Could you check a few things on this model? Use its own coordinates, in mm. Round coordinates to 2 decimals unless told otherwise and drop trailing zeros. Loops run counter-clockwise (first coordinate to the right, second up) from the corner with the lowest first, then second, coordinate; pieces in that order, holes last. Notation, with made-up numbers: (40.5, -29.75) -> (67.5, -29.75) arc R14 cw to (67.5, -4.75) -> close; hole circle Ø3 at (12, 40.5). An arc over 180 degrees is marked (long way). One line per item, written item: value.
Autodesk Inventor part; units mm, degrees
ref_plane "Startebene" through (0, 0, 0) normal (0, 0, 1) x (1, 0, 0)
ref_plane "Endebene" through (0, 0, 320) normal (0, 0, 1) x (1, 0, 0)
ref_plane "Startebene1" through (0, 0, 0) normal (0, 0, 1) x (1, 0, 0)
ref_plane "Startebene" through (0, 0, 0) normal (0, 0, 1) x (1, 0, 0)
ref_plane "Endebene" through (0, 0, 320) normal (0, 0, 1) x (1, 0, 0)
ref_plane "Startebene1" through (0, 0, 0) normal (0, 0, 1) x (1, 0, 0)
ref_plane "Endebene1" through (0, 0, 80) normal (0, 0, 1) x (1, 0, 0)
ref_plane "Startebene2" through (0, 0, 10) normal (0, 0, 1) x (1, 0, 0)
ref_plane "Endebene2" through (0, 0, 70) normal (0, 0, 1) x (1, 0, 0)
sketch "Skizze" plane through (0, 0, 0) normal (0, 0, 1) x (1, 0, 0)
  line L0 (-10, 9) -> (-10, 3.3)
  arc A0 (-10, 3.3) -> (-9.7, 3) centre (-9.7, 3.3) ccw
  line L1 (-9.7, 3) -> (-8, 3)
  line L2 (-8, 3) -> (-8, 6)
  line L3 (-8, 6) -> (-7.0607, 6)
  line L4 (-7.0607, 6) -> (-4, 2.9393)
  line L5 (-4, 2.9393) -> (-4, 0.3)
  line L6 (-4, 0.3) -> (-3.7, 0)
  line L7 (-3.7, 0) -> (-4, -0.3)
  line L8 (-4, -0.3) -> (-4, -2.9393)
  line L9 (-4, -2.9393) -> (-7.0607, -6)
  line L10 (-7.0607, -6) -> (-8, -6)
  line L11 (-8, -6) -> (-8, -3)
  line L12 (-8, -3) -> (-9.7, -3)
  arc A1 (-9.7, -3) -> (-10, -3.3) centre (-9.7, -3.3) ccw
  line L13 (-10, -3.3) -> (-10, -9)
  arc A2 (-10, -9) -> (-9, -10) centre (-9, -9) ccw
  line L14 (-9, -10) -> (-3.3, -10)
  arc A3 (-3.3, -10) -> (-3, -9.7) centre (-3.3, -9.7) ccw
  line L15 (-3, -9.7) -> (-3, -8)
  line L16 (-3, -8) -> (-6, -8)
  line L17 (-6, -8) -> (-6, -7.0607)
  line L18 (-6, -7.0607) -> (-2.9393, -4)
  line L19 (-2.9393, -4) -> (-0.3, -4)
  line L20 (-0.3, -4) -> (0, -3.7)
  line L21 (0, -3.7) -> (0.3, -4)
  line L22 (0.3, -4) -> (2.9393, -4)
  line L23 (2.9393, -4) -> (6, -7.0607)
  line L24 (6, -7.0607) -> (6, -8)
  line L25 (6, -8) -> (3, -8)
  line L26 (3, -8) -> (3, -9.7)
  arc A4 (3, -9.7) -> (3.3, -10) centre (3.3, -9.7) ccw
  line L27 (3.3, -10) -> (9, -10)
  arc A5 (9, -10) -> (10, -9) centre (9, -9) ccw
  line L28 (10, -9) -> (10, -3.3)
  arc A6 (10, -3.3) -> (9.7, -3) centre (9.7, -3.3) ccw
  line L29 (9.7, -3) -> (8, -3)
  line L30 (8, -3) -> (8, -6)
  line L31 (8, -6) -> (7.0607, -6)
  line L32 (7.0607, -6) -> (4, -2.9393)
  line L33 (4, -2.9393) -> (4, -0.3)
  line L34 (4, -0.3) -> (3.7, 0)
  line L35 (3.7, 0) -> (4, 0.3)
  line L36 (4, 0.3) -> (4, 2.9393)
  line L37 (4, 2.9393) -> (7.0607, 6)
  line L38 (7.0607, 6) -> (8, 6)
  line L39 (8, 6) -> (8, 3)
  line L40 (8, 3) -> (9.7, 3)
  arc A7 (9.7, 3) -> (10, 3.3) centre (9.7, 3.3) ccw
  line L41 (10, 3.3) -> (10, 9)
  arc A8 (10, 9) -> (9, 10) centre (9, 9) ccw
  line L42 (9, 10) -> (3.3, 10)
  arc A9 (3.3, 10) -> (3, 9.7) centre (3.3, 9.7) ccw
  line L43 (3, 9.7) -> (3, 8)
  line L44 (3, 8) -> (6, 8)
  line L45 (6, 8) -> (6, 7.0607)
  line L46 (6, 7.0607) -> (2.9393, 4)
  line L47 (2.9393, 4) -> (0.3, 4)
  line L48 (0.3, 4) -> (0, 3.7)
  line L49 (0, 3.7) -> (-0.3, 4)
  line L50 (-0.3, 4) -> (-2.9393, 4)
  line L51 (-2.9393, 4) -> (-6, 7.0607)
  line L52 (-6, 7.0607) -> (-6, 8)
  line L53 (-6, 8) -> (-3, 8)
  line L54 (-3, 8) -> (-3, 9.7)
  arc A10 (-3, 9.7) -> (-3.3, 10) centre (-3.3, 9.7) ccw
  line L55 (-3.3, 10) -> (-9, 10)
  arc A11 (-9, 10) -> (-10, 9) centre (-9, 9) ccw
  circle A12 centre (0, 0) radius 2.75
  dimension "d2" = 5.5
  dimension "d3" = 10
  dimension "d4" = 10
  dimension "d5" = 5.7
  dimension "d6" = 5.7
  dimension "d7" = 1.7
  dimension "d8" = 3
  dimension "d9" = 0.3
  dimension "d10" = 90
  dimension "d11" = 45
  dimension "d12" = 45
  dimension "d13" = 45
  dimension "d14" = 90
  dimension "d15" = 90
  dimension "d16" = 45
  dimension "d17" = 45
  dimension "d18" = 45
  dimension "d19" = 45
  dimension "d20" = 90
  dimension "d21" = 90
  dimension "d22" = 45
  dimension "d23" = 45
  dimension "d24" = 90
  dimension "d25" = 90
  dimension "d26" = 90
  dimension "d27" = 90
  dimension "d28" = 90
  dimension "d29" = 90
  dimension "d30" = 90
  dimension "d31" = 90
  dimension "d32" = 90
  dimension "d33" = 90
  dimension "d34" = 90
  dimension "d35" = 90
  dimension "d36" = 90
  dimension "d37" = 90
  dimension "d38" = 90
  dimension "d39" = 4
  dimension "d40" = 6
  dimension "d41" = 13
  dimension "d42" = 14
  dimension "d43" = 16
  dimension "d44" = 18
  dimension "d45" = 3
  dimension "d46" = 9
  dimension "d47" = 7
  dimension "d48" = 1
  dimension "d49" = 7
  dimension "d50" = 1.5
  dimension "d51" = 1.8663
  dimension "d52" = 3.3663
  dimension "d53" = 1.5
  dimension "d54" = 1.8663
  dimension "d55" = 3.3663
  dimension "d56" = 4
  dimension "d57" = 10.8187
  dimension "d58" = 1.9092
  dimension "d59" = 5
  dimension "d60" = 13
  dimension "d61" = 13
  dimension "d62" = 16.0513
  dimension "d63" = 3.3234
  dimension "d64" = 14
  dimension "d65" = 12.685
extrude "Körper" add sketch "Skizze" along normal up to surface (60 mm away) from surface at 10
sketch "Skizze13" plane through (0, 0, 0) normal (0, 0, 1) x (1, 0, 0)
  line L0 (0, 0) -> (10, 0)
ref_plane "Arbeitsebene12" through (0, 0, 0) normal (0, -1, 0) x (1, 0, 0)
sketch "Skizze14" plane through (0, 0, 0) normal (0, -1, 0) x (1, 0, 0)
  line L0 (-2, 10) -> (12, 10)
  line L1 (-2, 70) -> (12, 70)
  dimension "d80" = 60
ref_plane "Arbeitsebene13" through (9, -80, 70) normal (0, 0, 1) x (1, 0, 0)
split "Trennen1" plane through (9, -80, 70) removes the side toward (0, 0, 1)
ref_plane "Arbeitsebene14" through (3.3, -80, 10) normal (0, 0, -1) x (-1, 0, 0)
split "Trennen2" plane through (3.3, -80, 10) removes the side toward (0, 0, -1)
equation "\"G_OFFSET_START\" = 0"
equation "\"G_OFFSET_END\" = 0"
equation "\"G_L\" = d80"
equation "\"G_OFFSET_START1\" = 0"
equation "\"G_OFFSET_END1\" = 0"
properties part number "Alu Profil 20x20 - AP2020" material "Aluminium 6061"
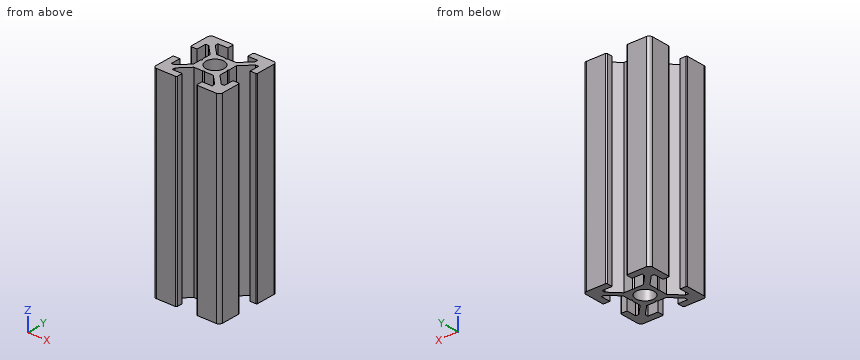
(1) If I drill on L1, parallel to Y at x = 8.5, z = 27.5; L2, parallel to Y at x = -5.25, z = 22.5; L3, parallel to X at y = -4.5, z = 25.5, over which ranges is the centre line in solid material (lowest first)?
Recorded:
L1: -10 to -3, 3 to 10
L2: -10 to -8, -6.31 to -4.19, 4.19 to 6.31, 8 to 10
L3: -10 to -8, -5.56 to -3.44, 3.44 to 5.56, 8 to 10
(2) I'm going to push flat-ended pins straight in: pin 1 Ø5 at (x, z) = (0, 20) entering from -Y; pin 2 Ø2 at (x, y) = (-0.5, 1.5) entering from -Z (3 decimals); pin 3 Ø2 at (y, z) = (1, 31.5) entering from -X. Where does each tip first touch, or does it pass through?
Recorded:
pin 1: y = -4
pin 2: through
pin 3: x = -4
(3) If we section it at A-A, the plane x = -2: Please give me the cut outline in (y, z).
Recorded:
outline: (-4, 10) -> (-1.89, 10) -> (-1.89, 70) -> (-4, 70) -> close; (1.89, 10) -> (4, 10) -> (4, 70) -> (1.89, 70) -> close
